Part model, mm, in its own coordinate system. Round coordinates to 2 decimals unless told otherwise and drop trailing zeros. Write each loop counter-clockwise with the first axis right and the second up, starting at its lowest first coordinate (ties: lowest second). Pieces come first, ordered by that corner, then holes. Notation, with made-up numbers: M -5,83.25 L 13,83.25 A27 cw 13,119.25 Z; hole C -1.5,4 d11. An arc over 180 degrees is marked long. One line per question, with ' | ' between items. Start each with the question number.
1) Saw through at A-A (z = 0.8). List the corners of the cut face in (x, y).
2) Wall check: probe 1 along Y at (x, z) = (-4.5, 0.4); probe 2 along X at (y, z) = (-21.5, 0.1). Give the ranges that are in metal, low to high. Write a range as [from, to].
3) Saw through at B-B (x = 11.5). List the corners of the cut face in (y, z), plus the area to 3 significant figures.
4) Drop a flat-ended pin along its axis: pin 1 Ø0.7 at (x, z) = (44.5, 0.5) entering from +Y. Give the stop position or say it passes through.
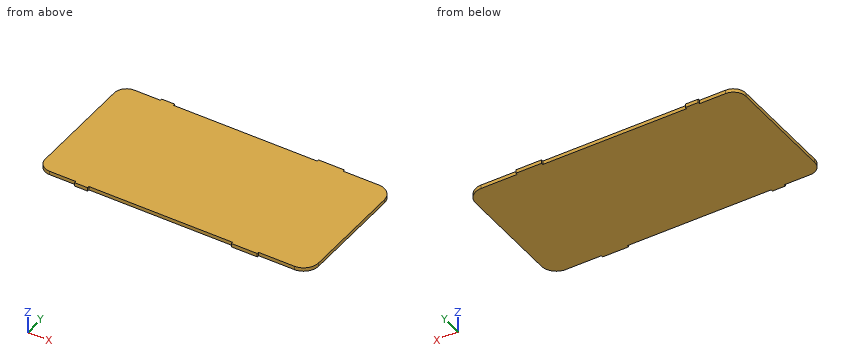
```python
from build123d import *

# Parameters (mm, degrees)
F0_W     = 55.6136657298
F0_H     = 51.5
F0_W_2   = 5
F0_W_3   = 10
F0_H_2   = 0.75
F1_DEPTH = 1.4


with BuildPart() as f1:
    # F0 (on Top) → F1 (new body)
    with BuildSketch(Plane.XY):
        with Locations((-3.5062433155, 0)):
            Rectangle(F0_W, F0_H)
        with Locations((-33.8130761804, 0)):
            Rectangle(F0_W_2, F0_H)
        with BuildLine():
            ThreePointArc((-51.2033691825, -21), (-49.8121263931, -24.3587572106), (-46.4533691825, -25.75))
            Line((-46.4533691825, -25.75), (-36.3130761804, -25.75))
            Line((-36.3130761804, -25.75), (-36.3130761804, 25.75))
            Line((-36.3130761804, 25.75), (-46.4533691825, 25.75))
            ThreePointArc((-46.4533691825, 25.75), (-49.8121263931, 24.3587572106), (-51.2033691825, 21))
            Line((-51.2033691825, 21), (-51.2033691825, -21))
        make_face()
        with Locations((29.3005895494, 0)):
            Rectangle(F0_W_3, F0_H)
        with BuildLine():
            Line((34.3005895494, 25.75), (34.3005895494, -25.75))
            Line((34.3005895494, -25.75), (48.1754575549, -25.75))
            ThreePointArc((48.1754575549, -25.75), (52.2413215467, -24.0658639918), (53.9254575549, -20))
            Line((53.9254575549, -20), (53.9254575549, 20))
            ThreePointArc((53.9254575549, 20), (52.2413215467, 24.0658639918), (48.1754575549, 25.75))
            Line((48.1754575549, 25.75), (34.3005895494, 25.75))
        make_face()
        with Locations((29.3005895494, -26.125)):
            Rectangle(F0_W_3, F0_H_2)
        with Locations((29.3005895494, 26.125)):
            Rectangle(F0_W_3, F0_H_2)
        with Locations((-33.8130761804, 26.125)):
            Rectangle(F0_W_2, F0_H_2)
        with Locations((-33.8130761804, -26.125)):
            Rectangle(F0_W_2, F0_H_2)
    extrude(amount=F1_DEPTH)


solid = f1.part
```
Answer key:
1) outline: M -51.2,-21 A4.75 ccw -46.45,-25.75 L -36.31,-25.75 L -36.31,-26.5 L -31.31,-26.5 L -31.31,-25.75 L 24.3,-25.75 L 24.3,-26.5 L 34.3,-26.5 L 34.3,-25.75 L 48.18,-25.75 A5.75 ccw 53.93,-20 L 53.93,20 A5.75 ccw 48.18,25.75 L 34.3,25.75 L 34.3,26.5 L 24.3,26.5 L 24.3,25.75 L -31.31,25.75 L -31.31,26.5 L -36.31,26.5 L -36.31,25.75 L -46.45,25.75 A4.75 ccw -51.2,21 Z
2) probe 1: y = [-25.75, 25.75] | probe 2: x = [-51.18, 53.73]
3) outline: M -25.75,0 L 25.75,0 L 25.75,1.4 L -25.75,1.4 Z | area: 72.1 mm2
4) pin 1: stops at y = 25.75
